```python
from build123d import *

# Parameters (mm, degrees)
F0_W      = 90
F0_H      = 90
F0_R      = 4
F1_DEPTH  = 10
F2_R      = 40
F2_R_2    = 38
F3_DEPTH  = 100
F7_SIZE   = 1
F8_SIZE   = 1
F10_R     = 4
F11_DEPTH = 80


with BuildPart() as f1:
    # F0 (on Top) → F1 (new body)
    with BuildSketch(Plane.XY):
        Rectangle(F0_W, F0_H)
        with Locations((-37, -37)):
            Circle(F0_R, mode=Mode.SUBTRACT)
        with Locations((37, -37)):
            Circle(F0_R, mode=Mode.SUBTRACT)
        with Locations((-37, 37)):
            Circle(F0_R, mode=Mode.SUBTRACT)
        with Locations((37, 37)):
            Circle(F0_R, mode=Mode.SUBTRACT)
    extrude(amount=-F1_DEPTH)

    # F2 (on face) → F3 (join)
    with BuildSketch(Plane.XY):
        Circle(F2_R)
        Circle(F2_R_2, mode=Mode.SUBTRACT)
    extrude(amount=F3_DEPTH)

    # F5 (on Front) → F6 (revolve)
    with BuildSketch(Plane.XZ):
        Polygon((0, 52), (0, 50), (22, 50), (22, 100), (40, 100), (40, 102), (20, 102), (20, 52), align=None)
    revolve(axis=Axis((0, 0, 75.148744), (0, 0, 1)))

    # F7
    f7_edges = [f1.edges().sort_by_distance(p)[0] for p in [
        (-40, 0, 0),
        (40, 0, 51),
        (-40, 0, 102),
    ]]
    chamfer(f7_edges, length=F7_SIZE)

    # F8
    f8_edges = [f1.edges().sort_by_distance(p)[0] for p in [
        (-20, 0, 102),
    ]]
    chamfer(f8_edges, length=F8_SIZE)

    # F10 (on offset) → F11 (cut)
    with BuildSketch(Plane.XZ.offset(40)):
        with Locations((0, 77)):
            Circle(F10_R)
    extrude(amount=-F11_DEPTH, mode=Mode.SUBTRACT)


solid = f1.part
```
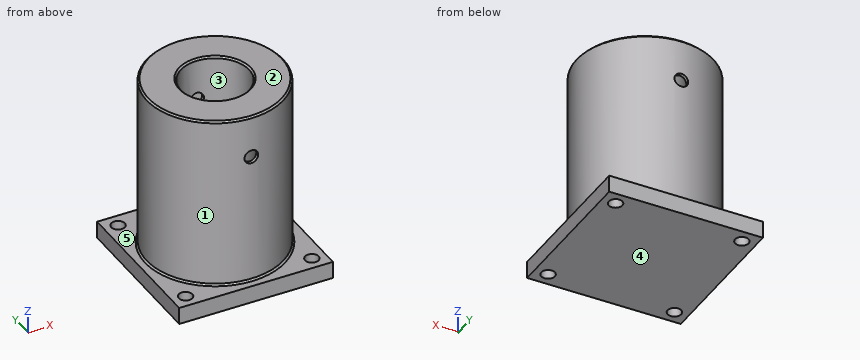
Input: part model. Units: mm. Frame: model coordinates. Face numbers are marked on the shaded views. A direction names the side the tool comes from. Give positions to 0.01 mm unless a question says otherwise; leave off trailing zeros. Order: outer loops, then holes, each group sorted by start corner. A loop starts at its lowest first (then second) coordinate and runs counter-clockwise, first axis right, second up.
1. Pin query (flat end, axial travel): pin 1 (10 mm diameter, centred on x = 34, z = 73, fed in from +Y); pin 2 (6 mm diameter, centred on x = 12.5, z = 86.5, fed in from +Y); pin 3 (6 mm diameter, centred on y = -3.5, z = 86.5, fed in from +X). Return the tip coordinate at first contact, or that it passes through.
Derived:
pin 1: stops at y = 27.55
pin 2: stops at y = 38.86
pin 3: stops at x = 40
2. Section C-C on x = 0. Give the number of separate pieces and of enclosed holes in the cut face, and give its area (4 significant figures).
Derived:
separate pieces: 4
enclosed holes: 0
area: 1,595 mm2
3. Section A-A on y = 0. Return the cut outline in (x, z), and give its area (3 significant figures).
Derived:
outline: (-45, -10) - (45, -10) - (45, 0) - (41, 0) - (40, 1) - (40, 101) - (39, 102) - (21, 102) - (20, 101) - (20, 52) - (-20, 52) - (-20, 101) - (-21, 102) - (-39, 102) - (-40, 101) - (-40, 1) - (-41, 0) - (-45, 0) - close; hole (-38, 0) - (38, 0) - (38, 100) - (22, 100) - (22, 50) - (-22, 50) - (-22, 100) - (-38, 100) - close
area: 1,660 mm2
4. Reachability of the marked faces 4 and 5 from +Z, -Z, +X, -X, +Y, -Y: full face, straight path, thin tool, end or side. Return the list, or none.
Derived:
face 4: -Z, +X, -X, +Y, -Y
face 5: +Z
5. Section B-B on z = 63.5. Return the cut outline in (x, y).
Derived:
outline: circle Ø80 at (0, 0); circle Ø44 at (0, 0); hole circle Ø76 at (0, 0); hole circle Ø40 at (0, 0)
6. Section D-D on z = 46. Return the cut outline in (x, y).
Derived:
outline: circle Ø80 at (0, 0); hole circle Ø76 at (0, 0)
7. Material intervals for L1, parallel to Y at x = 37, z = -3.75; L2, parallel to Z at x = 0, y = -15.5; L3, parallel to Z at x = 7, y = -37, sorted ascending.
Derived:
L1: y = -45 to -41, -33 to 33, 41 to 45
L2: z = -10 to 0, 50 to 52
L3: z = -10 to 0, 100 to 102
8. Mould query, pull axis X, two halves, no side actions, for the marked faces 1, 2 and 3. Classes: released by +X, released by -X, zero draft, split by the parting line, or undercut.
Derived:
face 1: split by the parting line
face 2: zero draft
face 3: undercut
